Can you work these out from the model? Positions are in its coordinate system, mm. Face numbers are marked on the shaded views. A direction names the side the tool comes from. Coordinates: 2 decimals unless noted, no trailing zeros. Order: outer loops, then holes, each group sorted by start corner. A loop starts at its lowest first (then second) coordinate and runs counter-clockwise, first axis right, second up. Notation, with made-up numbers: (24.5, 75) - (37.5, 75) arc R11 cw to (37.5, 86) - close; hole circle Ø7 at (64, 50.25). An arc over 180 degrees is marked (long way). Use a Markdown table: item, result. Add a question column.
(1) I want a section at C-C (x = 0). List the corners of the cut face in (y, z) for me, and give its area (3 significant figures).
(2) We'd pull the mould along Y, two halves only. Please class the marked faces 3, 4 and 5: pulls with the +Y half, pulls with the -Y half, needs draft (parallel to the pull), parting line crosses it, or undercut.
(3) I want a section at B-B (z = 12.5). List the corners of the cut face in (x, y) for me.
(4) I want a section at D-D (y = 2.5). List the corners of the cut face in (x, z) for me.
(5) If I drill on L1, parallel to Y at x = 0, z = 6.5; L2, parallel to X at y = 0.75, z = 5.5; L3, parallel to Z at x = -2.5, y = 0, over which ranges is the centre line in solid material (lowest first)? Write a range as [from, to].
(6) For pin 1 Ø3 at (x, z) = (0, 6) entering from +Y; pin 2 Ø4 at (x, y) = (-0.5, 2.5) entering from -Z, each with a flat end and sliding along its axis, tell me the tip position at first contact or that it passes through.
(7) I want a section at A-A (z = 9). List the corners of the cut face in (x, y) for me.
(8) On a 3-axis mill with a long thin cutter (end or side, diameter ignored), from which of +Z, -Z, +X, -X, +Y, -Y can I reach the whole of each face in a straight line? I mean the marked faces 1 and 2. Say none if no direction works.
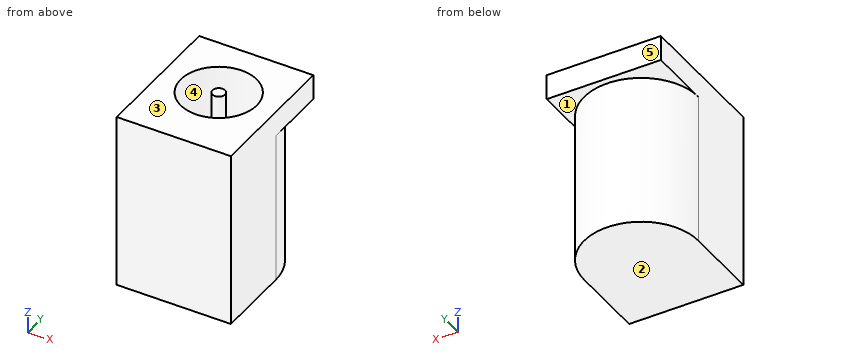
```python
from build123d import *

# Parameters (mm, degrees)
SKETCH1_W           = 9
SKETCH1_H           = 11
BOSS_EXTRUDE1_DEPTH = 14
SKETCH2_R           = 3
CUT_EXTRUDE1_DEPTH  = 12
SKETCH3_OUTSIDE_W   = 14.99
SKETCH3_OUTSIDE_H   = 16.99
CUT_EXTRUDE2_DEPTH  = 12
SKETCH4_R           = 1
BOSS_EXTRUDE2_DEPTH = 2
SKETCH5_R           = 0.5
BOSS_EXTRUDE3_DEPTH = 10


with BuildPart() as part:
    # Sketch1 → Boss-Extrude1 (new body)
    with BuildSketch(Plane.XY):
        Rectangle(SKETCH1_W, SKETCH1_H)
    extrude(amount=BOSS_EXTRUDE1_DEPTH)

    # Sketch2 → Cut-Extrude1 (cut)
    with BuildSketch(Plane.XY.offset(14)):
        with Locations((0, 0.5)):
            Circle(SKETCH2_R)
    extrude(amount=-CUT_EXTRUDE1_DEPTH, mode=Mode.SUBTRACT)

    # Sketch3 outside → Cut-Extrude2 (cut)
    with BuildSketch(Plane(origin=(0, 0, 0), x_dir=(-1, 0, 0), z_dir=(0, 0, -1))):
        Rectangle(SKETCH3_OUTSIDE_W, SKETCH3_OUTSIDE_H)
        with BuildLine():
            Line((-4.5, 0.5), (-4.5, -5.5))
            Line((-4.5, -5.5), (4.5, -5.5))
            Line((4.5, -5.5), (4.5, 0.5))
            ThreePointArc((4.5, 0.5), (0, 5), (-4.5, 0.5))
        make_face(mode=Mode.SUBTRACT)
    extrude(amount=-CUT_EXTRUDE2_DEPTH, mode=Mode.SUBTRACT)

    # Sketch4 → Boss-Extrude2 (add)
    with BuildSketch(Plane.XY.offset(2)):
        with Locations((0, 0.5)):
            Circle(SKETCH4_R)
    extrude(amount=BOSS_EXTRUDE2_DEPTH)

    # Sketch5 → Boss-Extrude3 (add)
    with BuildSketch(Plane.XY.offset(4)):
        with Locations((0, 0.5)):
            Circle(SKETCH5_R)
    extrude(amount=BOSS_EXTRUDE3_DEPTH)


solid = part.part
```
Answers follow:
| question | item | result |
|---|---|---|
| 1 | outline | (-5.5, 0) - (5, 0) - (5, 12) - (5.5, 12) - (5.5, 14) - (3.5, 14) - (3.5, 2) - (1.5, 2) - (1.5, 4) - (1, 4) - (1, 14) - (0, 14) - (0, 4) - (-0.5, 4) - (-0.5, 2) - (-2.5, 2) - (-2.5, 14) - (-5.5, 14) - close |
| 1 | area | 90.0 mm² |
| 2 | face 3 | needs draft |
| 2 | face 4 | undercut |
| 2 | face 5 | pulls with the +Y half |
| 3 | outline | (-4.5, -5.5) - (4.5, -5.5) - (4.5, 5.5) - (-4.5, 5.5) - close; circle Ø1 at (0, 0.5); hole circle Ø6 at (0, 0.5) |
| 4 | outline | (-4.5, 12) - (-4.03, 12) - (-4.03, 0) - (4.03, 0) - (4.03, 12) - (4.5, 12) - (4.5, 14) - (2.24, 14) - (2.24, 2) - (-2.24, 2) - (-2.24, 14) - (-4.5, 14) - close |
| 5 | L1 | y = [-5.5, -2.5], [0, 1], [3.5, 5] |
| 5 | L2 | x = [-4.49, -2.99], [-0.43, 0.43], [2.99, 4.49] |
| 5 | L3 | z = [0, 2] |
| 6 | pin 1 | stops at y = 5 |
| 6 | pin 2 | stops at z = 0 |
| 7 | outline | (-4.5, -5.5) - (4.5, -5.5) - (4.5, 0.5) arc R4.5 ccw to (-4.5, 0.5) - close; circle Ø1 at (0, 0.5); hole circle Ø6 at (0, 0.5) |
| 8 | face 1 | -Z, +Y |
| 8 | face 2 | -Z, +X, -X, +Y, -Y |
